```python
from build123d import *

# Parameters (mm, degrees)
SKETCH2_R           = 17.907
BOSS_EXTRUDE1_DEPTH = 69.85
SKETCH3_R           = 3.175
BOSS_EXTRUDE2_DEPTH = 49.53
SKETCH4_R           = 17.907
CUT_EXTRUDE1_DEPTH  = 2.54


with BuildPart() as part:
    # Sketch2 → Boss-Extrude1 (new body)
    with BuildSketch(Plane(origin=(0, 0, 0), x_dir=(1, 0, 0), z_dir=(0, 1, 0))):
        with Locations(Location((0, 0, 0), (0, 0, 270))):
            Circle(SKETCH2_R)
    extrude(amount=BOSS_EXTRUDE1_DEPTH)

    # Sketch3 → Boss-Extrude2 (add)
    with BuildSketch(Plane.XY):
        with Locations(Location((0, 6.35, 0), (0, 0, 180))):
            Circle(SKETCH3_R)
    extrude(amount=BOSS_EXTRUDE2_DEPTH)

    # Sketch4 → Cut-Extrude1 (cut)
    with BuildSketch(Plane.XZ):
        with Locations(Location((0, 0, 0), (0, 0, 270))):
            Circle(SKETCH4_R)
    extrude(amount=-CUT_EXTRUDE1_DEPTH, mode=Mode.SUBTRACT)


solid = part.part
```
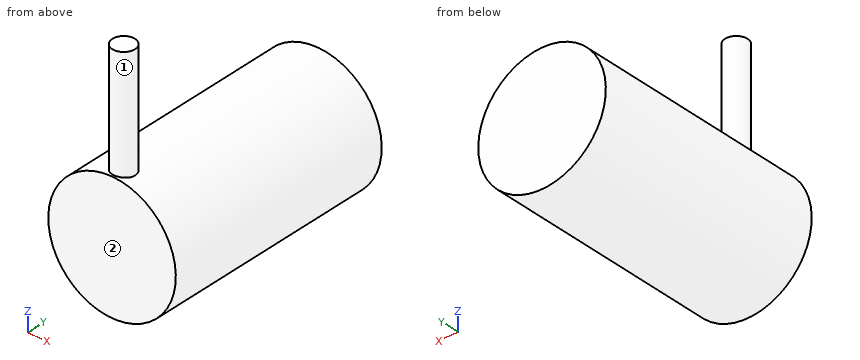
Can you work these out from the model? Positions are in its coordinate system, mm. Face numbers are marked on the shaded views. A direction names the side the tool comes from. Round coordinates to 2 decimals unless told otherwise and drop trailing zeros. Order: outer loops, then holes, each group sorted by start corner. A loop starts at its lowest first (then second) coordinate and runs counter-clockwise, first axis right, second up. Notation, with made-up numbers: (68.25, 13.25) -> (123.25, 13.25) arc R28 ccw to (123.25, 31.25) -> close; hole circle Ø3 at (46.25, 73). An arc over 180 degrees is marked (long way). Return JSON: item names as keys, results as strings. Group by question number.
1. If we section it at A-A, the plane x = 0: Write out the boundary of the cut face in (y, z) (3 decimals).
2. I need wall thicknesses on line 1 (Z direction, x = -1, y = 31); line 2 (Z direction, x = 7.5, y = 37); line 3 (X direction, y = 12.5, z = -4.5). Which ranges of each line are inside material? Lowest first, please. Write a range as [from, to].
3. If we section it at B-B, the plane y = 6.35: Write out the boundary of the cut face in (x, z) (3 decimals), then the cut area to 3 significant figures.
4. If we section it at D-D, the plane y = 17: Write out the boundary of the cut face in (x, z).
5. Which directions (+Z, -Z, +X, -X, +Y, -Y) give clear straight access to the entire face, cutting with the end or side of a thin tool? Please do the marked faces 1 and 2.
6. Will these pins go through, and if not, where does the flat tip stop? pin 1 (1 mm diameter, centred on x = -2, y = 9.5, fed in from +Z); pin 2 (4 mm diameter, centred on x = 6, y = 49.5, fed in from +Z); pin 3 (10 mm diameter, centred on y = 42.5, z = 1, fed in from +X).
7. If we section it at C-C, the plane z = 35: Write out the boundary of the cut face in (x, y) (3 decimals).
Output values:
{
 "1": {"outline": "(2.54, -17.907) -> (69.85, -17.907) -> (69.85, 17.907) -> (9.525, 17.907) -> (9.525, 49.53) -> (3.175, 49.53) -> (3.175, 17.907) -> (2.54, 17.907) -> close"},
 "2": {"line 1": "[-17.88, 17.88]", "line 2": "[-16.26, 16.26]", "line 3": "[-17.33, 17.33]"},
 "3": {"outline": "(-3.175, 17.623) arc R17.907 ccw (long way) to (3.175, 17.623) -> (3.175, 49.53) -> (-3.175, 49.53) -> close", "area": "1,210 mm²"},
 "4": {"outline": "circle Ø35.81 at (0, 0)"},
 "5": {"face 1": "+Z", "face 2": "+Z, -Z, +X, -X, -Y"},
 "6": {"pin 1": "z = 17.84", "pin 2": "z = 17.45", "pin 3": "x = 17.91"},
 "7": {"outline": "circle Ø6.35 at (0, 6.35)"}
}
